```python
from build123d import *

# Parameters (mm, degrees)
SKETCH_1_R             = 23.5
EXTRUDE_1_DEPTH        = 8
SKETCH_2_W             = 16
SKETCH_2_H             = 5
EXTRUDE_2_DEPTH        = 70
FILLET_2_R             = 1
HOLE_WIZARD_M6_1_D     = 5
HOLE_WIZARD_M6_1_DEPTH = 7
HOLE_WIZARD_M6_1_TIP   = 1.502151548


with BuildPart() as part:
    # 草图1 → 凸台-拉伸1 (new body)
    with BuildSketch(Plane.XY):
        Polygon((30, -32.5), (-30, -32.5), (-30, 0), (-30, 35), (30, 35), align=None)
        Circle(SKETCH_1_R, mode=Mode.SUBTRACT)
    extrude(amount=EXTRUDE_1_DEPTH)

    # 草图2 → 凸台-拉伸2 (add)
    with BuildSketch(Plane(origin=(30, 0, 0), x_dir=(0, 0, -1), z_dir=(1, 0, 0))):
        with Locations((-4, -30)):
            Rectangle(SKETCH_2_W, SKETCH_2_H)
    extrude_2 = extrude(amount=-EXTRUDE_2_DEPTH)

    # 镜向1: 凸台-拉伸2 across plane
    add(extrude_2.mirror(Plane.ZY))

    # 圆角2
    fillet_2_edges = [part.edges().sort_by_distance(p)[0] for p in [
        (0, -27.5, 0),
        (-40, -27.5, 4),
        (0, -27.5, 12),
        (-30, -27.5, 4),
        (0, -27.5, 8),
        (0, -27.5, -4),
        (30, -27.5, 4),
        (40, -27.5, 4),
    ]]
    fillet(fillet_2_edges, radius=FILLET_2_R)

    # M6 螺纹孔1
    with Locations(Plane(origin=(0, 35, 0), x_dir=(1, 0, 0), z_dir=(0, 1, 0))):
        with Locations((-20, -4), (20, -4)):
            Hole(HOLE_WIZARD_M6_1_D / 2, depth=HOLE_WIZARD_M6_1_DEPTH)
            with Locations((0, 0, -(HOLE_WIZARD_M6_1_DEPTH + HOLE_WIZARD_M6_1_TIP / 2))):  # 118° drill point
                Cone(0, HOLE_WIZARD_M6_1_D / 2, HOLE_WIZARD_M6_1_TIP, mode=Mode.SUBTRACT)


solid = part.part
```
The listing builds one solid part. Answer for the finished solid, in the listing's coordinates (mm). A direction names the side the tool comes from. Give positions to 0.01 mm unless a question says otherwise; leave off trailing zeros. Order: outer loops, then holes, each group sorted by start corner. A loop starts at its lowest first (then second) coordinate and runs counter-clockwise, first axis right, second up. Notation, with made-up numbers: (27.25, 58.25) - (55.25, 58.25) arc R9 ccw to (55.25, 73.25) - close; hole circle Ø7 at (2, 19.25). An arc over 180 degrees is marked (long way). Answer in a Markdown table with one row per item. Add a question column.
Q1. Which of the six approach directions +Z, -Z, +X, -X, +Y, -Y give full straight-line access (tool end or side, diameter ignored) to faces 1 (the flat face through (30, 5, 4)), 2 (the flat face through (-1, -31, 12)), 3 (the cylindrical face through (-17.5, 31.5, 3.9)), 4 (the flat face through (-40, -30, 4)), 5 (the flat face through (0, 25, 0))?
Q2. The part is cut by section B-B (x = 0). Determine the outline of the cut face in (y, z).
Q3. Find the intervals of material crossed by line 1 along Y through (x, z) = (0, 2); line 2 along Z through (x, y) = (-20, 32); line 3 along Y through (x, z) = (-22, -1.75), in increasing order. Write a range as [from, to].
Q4. The part is cut by section A-A (y = 0). Determine the outline of the cut face in (x, z).
Q5. For a pull along X with two mould halves and no side action, classify faces 6 (the flat face through (0, 25, 8)), 7 (the flat face through (-30, 5, 4)), 8 (the conical face through (19.68, 26.759, 3.707)) as released by +X, released by -X, zero draft, split by the parting line, or undercut.
Q6. The part is cut by section D-D (y = -25.5). Determine the outline of the cut face in (x, z), then the cut area to 3 significant figures.
Q7. The part is cut by section C-C (x = -28). Determine the outline of the cut face in (y, z), then the cut area to 3 significant figures.
Q8. Given P1, Ø6, axis at y = -10.5, z = 5, coming from the +X side; P2, Ø3, axis at y = 1, z = 9, coming from the -X side; P3, Ø4.5, axis at x = -20, z = 4, coming from the +Y side, each flat-ended and moving along its own axis, determine where each tip first touches the part or whether it passes through.
Determined:
| question | item | result |
|---|---|---|
| 1 | face 1 | +Z, -Z, +X, +Y |
| 1 | face 2 | +Z, +X, -X, +Y, -Y |
| 1 | face 3 | +Y |
| 1 | face 4 | +Z, -Z, -X, +Y, -Y |
| 1 | face 5 | -Z, +X, -X, +Y |
| 2 | outline | (-32.5, -4) - (-28.5, -4) arc R1 ccw to (-27.5, -3) - (-27.5, -1) arc R1 cw to (-26.5, 0) - (-23.5, 0) - (-23.5, 8) - (-26.5, 8) arc R1 cw to (-27.5, 9) - (-27.5, 11) arc R1 ccw to (-28.5, 12) - (-32.5, 12) - close; (23.5, 0) - (35, 0) - (35, 8) - (23.5, 8) - close |
| 3 | line 1 | y = [-32.5, -23.5], [23.5, 35] |
| 3 | line 2 | z = [0, 1.5], [6.5, 8] |
| 3 | line 3 | y = [-32.5, -27.5] |
| 4 | outline | (-30, 0) - (-23.5, 0) - (-23.5, 8) - (-30, 8) - close; (23.5, 0) - (30, 0) - (30, 8) - (23.5, 8) - close |
| 5 | face 6 | zero draft |
| 5 | face 7 | released by -X |
| 5 | face 8 | undercut |
| 6 | outline | (-30, 0) - (30, 0) - (30, 8) - (-30, 8) - close |
| 6 | area | 480 mm² |
| 7 | outline | (-32.5, -4) - (-28.5, -4) arc R1 ccw to (-27.5, -3) - (-27.5, -1) arc R1 cw to (-26.5, 0) - (35, 0) - (35, 8) - (-26.5, 8) arc R1 cw to (-27.5, 9) - (-27.5, 11) arc R1 ccw to (-28.5, 12) - (-32.5, 12) - close |
| 7 | area | 580 mm² |
| 8 | P1 | stops at x = 30 |
| 8 | P2 | stops at x = -30 |
| 8 | P3 | stops at y = 27.85 |
